The listing builds one solid part. Answer for the finished solid, in the listing's coordinates (mm). A direction names the side the tool comes from. Coordinates: 2 decimals unless noted, no trailing zeros. Write each loop counter-clockwise with the first axis right and the second up, starting at its lowest first coordinate (ties: lowest second). Pieces come first, ordered by that corner, then holes.
from build123d import *

# Parameters (mm, degrees)
SKETCH_1_R                   = 12
EXTRUDE_894_DEPTH            = 30
HOLE_WIZARD_5_D              = 4.2
HOLE_WIZARD_5_CSINK_D        = 5.05
HOLE_WIZARD_5_CSINK_ANGLE    = 90
PATTERN_CIRCULAR_1906_COUNT  = 8
SKETCH_27_W                  = 19
SKETCH_27_H                  = 30
CUT_EXTRUDE_2273_DEPTH       = 1
HOLE_WIZARD_2331_D           = 4.2
HOLE_WIZARD_2331_DEPTH       = 15
HOLE_WIZARD_2331_CSINK_D     = 5.05
HOLE_WIZARD_2331_CSINK_ANGLE = 90
HOLE_WIZARD_2331_TIP         = 1.2618073


with BuildPart() as part:
    # Эскиз1 → Extrude 894 (new body)
    with BuildSketch(Plane.XY):
        Polygon((-22.5, 18), (0, 18), (22.5, 18), (22.5, -6), (14, -18), (-14, -18), (-22.5, -6), align=None)
        Circle(SKETCH_1_R, mode=Mode.SUBTRACT)
    extrude(amount=-EXTRUDE_894_DEPTH)

    # Гайка М5 (through all)
    with Locations(Plane.XY):
        with Locations((-16, 0)):
            hole_wizard_5 = CounterSinkHole(HOLE_WIZARD_5_D / 2, HOLE_WIZARD_5_CSINK_D / 2, counter_sink_angle=HOLE_WIZARD_5_CSINK_ANGLE)

    # Pattern Circular 1906: Гайка М5 ×8 about axis, 2 skipped
    pattern_circular_1906_axis = Axis((0, 0, 0), (0, 0, 1))
    add([hole_wizard_5.rotate(pattern_circular_1906_axis, i * 360 / PATTERN_CIRCULAR_1906_COUNT) for i in range(1, PATTERN_CIRCULAR_1906_COUNT) if i not in (2, 6)], mode=Mode.SUBTRACT)

    # Эскиз27 → Cut-Extrude 2273 (cut)
    with BuildSketch(Plane(origin=(0, 18, 0), x_dir=(1, 0, 0), z_dir=(0, 1, 0))):
        with Locations((0, 15)):
            Rectangle(SKETCH_27_W, SKETCH_27_H)
    extrude(amount=-CUT_EXTRUDE_2273_DEPTH, mode=Mode.SUBTRACT)

    # Hole Wizard 2331
    with Locations(Plane(origin=(0, 18, 0), x_dir=(1, 0, 0), z_dir=(0, 1, 0))):
        with Locations((16, 15), (-16, 15)):
            CounterSinkHole(HOLE_WIZARD_2331_D / 2, HOLE_WIZARD_2331_CSINK_D / 2, depth=HOLE_WIZARD_2331_DEPTH, counter_sink_angle=HOLE_WIZARD_2331_CSINK_ANGLE)
            with Locations((0, 0, -(HOLE_WIZARD_2331_DEPTH + HOLE_WIZARD_2331_TIP / 2))):  # 118° drill point
                Cone(0, HOLE_WIZARD_2331_D / 2, HOLE_WIZARD_2331_TIP, mode=Mode.SUBTRACT)


solid = part.part
Q1. The part is cut by section B-B, the plane y = 5.5. Write down the section's boundary in (x, z), then the cut area to 3 significant figures.
Answers below:
outline: (-22.5, -30) - (-10.67, -30) - (-10.67, 0) - (-22.5, 0) - close; (10.67, -30) - (22.5, -30) - (22.5, 0) - (10.67, 0) - close; hole circle Ø4.2 at (-16, -15); hole circle Ø4.2 at (16, -15)
area: 682 mm2
Q2. The part is cut by section C-C, the plane z = -15. State how many separate pieces and enclosed holes the cut face has, then the cut area to 3 significant figures.
Answers below:
separate pieces: 1
enclosed holes: 5
area: 832 mm2
Q3. The part is cut by section D-D, the plane x = -2. Write down the section's boundary in (y, z).
Answers below:
outline: (-18, -30) - (-11.83, -30) - (-11.83, 0) - (-18, 0) - close; (11.83, -30) - (17, -30) - (17, 0) - (11.83, 0) - close
Q4. Given pin 1 (5.5 mm diameter, centred on x = -16, z = -15, fed in from -Y); pin 2 (5 mm diameter, centred on x = -16, y = 0, fed in from +Z) (3 decimals); pin 3 (1.5 mm diameter, centred on y = -9.5, z = -25.5, fed in from +X); pin 4 (5 mm diameter, centred on x = 16, z = -15, fed in from +Y) (3 decimals), each flat-ended and moving along its own axis, determine where each tip first touches the part or whether it passes through.
Answers below:
pin 1: stops at y = -18
pin 2: stops at z = -0.025
pin 3: stops at x = 20.55
pin 4: stops at y = 17.975
Q5. The part is cut by section A-A, the plane y = 0. Write down the section's boundary in (x, z) (3 decimals).
Answers below:
outline: (-22.5, -30) - (-18.1, -30) - (-18.1, -0.425) - (-18.525, 0) - (-22.5, 0) - close; (-13.9, -30) - (-12, -30) - (-12, 0) - (-13.475, 0) - (-13.9, -0.425) - close; (12, -30) - (13.9, -30) - (13.9, -0.425) - (13.475, 0) - (12, 0) - close; (18.1, -30) - (22.5, -30) - (22.5, 0) - (18.525, 0) - (18.1, -0.425) - close
Q6. Which of the six approach directions +Z, -Z, +X, -X, +Y, -Y give full straight-line access (tool end or side, diameter ignored) to faces 5 (the face through (12.117, 13.254, -15.42)), 6 (the face through (-17.13, 10.19, -16.77))?
Answers below:
face 5: +Z, -Z
face 6: +Y
Q7. Find the intervals of material crossed by probe 1 along Y at (x, z) = (0.5, -2.5); probe 2 along X at (y, z) = (-1.5, -22); probe 3 along X at (y, z) = (2.5, -14.5), in increasing order.
Answers below:
probe 1: y = -18 to -11.99, 11.99 to 17
probe 2: x = -22.5 to -17.47, -14.53 to -11.91, 11.91 to 14.53, 17.47 to 22.5
probe 3: x = -22.5 to -17.17, -14.83 to -11.74, 11.74 to 14.83, 17.17 to 22.5
Q8. Determine the mould class of faces 1 (the face through (-22.5, 6, -15)), 2 (the face through (18.31, -11.916, -14.79)), 3 (the face through (9.5, 17.5, -14.8)), 4 (the face through (-16.969, -1.863, -15.42)) for opening direction X: released by +X, released by -X, zero draft, split by the parting line, or undercut.
Answers below:
face 1: released by -X
face 2: released by +X
face 3: undercut
face 4: undercut
